```python
from build123d import *

# Parameters (mm, degrees)
SKETCH1_W           = 49.1
SKETCH1_H           = 80
BOSS_EXTRUDE1_DEPTH = 2
SKETCH2_R           = 1.7
CUT_EXTRUDE1_DEPTH  = 2
SKETCH3_W           = 5.2
SKETCH3_H           = 5.2
SKETCH3_R           = 1.7
BOSS_EXTRUDE2_DEPTH = 3.3
SKETCH4_W           = 7.5
SKETCH4_H           = 17.15
SKETCH4_W_2         = 5.1
CUT_EXTRUDE2_DEPTH  = 3.3
SKETCH7_W           = 38.7
SKETCH7_H           = 2.4
SKETCH7_W_2         = 2.4
SKETCH7_H_2         = 45.05
BOSS_EXTRUDE4_DEPTH = 3.3
SKETCH8_W           = 6.6
SKETCH8_H           = 1.2
SKETCH8_W_2         = 4.7
SKETCH8_H_2         = 6.2
BOSS_EXTRUDE5_DEPTH = 2.4
FILLET1_START       = -9.5
FILLET1_DEPTH       = 12.5
SKETCH9_R           = 2.5
CUT_EXTRUDE3_DEPTH  = 2
FILLET2_R           = 0.2


with BuildPart() as part:
    # Sketch1 → Boss-Extrude1 (new body)
    with BuildSketch(Plane(origin=(0, 0, 0), x_dir=(1, 0, 0), z_dir=(0, 1, 0))):
        with Locations((24.55, -40)):
            Rectangle(SKETCH1_W, SKETCH1_H)
    extrude(amount=BOSS_EXTRUDE1_DEPTH)

    # Sketch2 → Cut-Extrude1 (cut)
    with BuildSketch(Plane(origin=(0, 2, 0), x_dir=(1, 0, 0), z_dir=(0, 1, 0))):
        with Locations(Location((2.4, -77.6, 0), (0, 0, 270))):
            Circle(SKETCH2_R)
        with Locations(Location((2.45, -26.95, 0), (0, 0, 270))):
            Circle(SKETCH2_R)
        with Locations(Location((2.45, -5, 0), (0, 0, 270))):
            Circle(SKETCH2_R)
        with Locations(Location((46.7, -77.6, 0), (0, 0, 90))):
            Circle(SKETCH2_R)
        with Locations(Location((46.65, -26.95, 0), (0, 0, 90))):
            Circle(SKETCH2_R)
        with Locations(Location((46.65, -5, 0), (0, 0, 90))):
            Circle(SKETCH2_R)
    extrude(amount=-CUT_EXTRUDE1_DEPTH, mode=Mode.SUBTRACT)

    # Sketch3 → Boss-Extrude2 (add)
    # profile 1 of 6: a face of its own
    with BuildSketch(Plane.XZ):
        with Locations((2.6, 77.4)):
            Rectangle(SKETCH3_W, SKETCH3_H)
        with Locations(Location((2.4, 77.6, 0), (0, 0, 90))):
            Circle(SKETCH3_R, mode=Mode.SUBTRACT)
    # profile 2 of 6: a face of its own
    with BuildSketch(Plane.XZ):
        with Locations((2.6, 27.15)):
            Rectangle(SKETCH3_W, SKETCH3_H)
        with Locations(Location((2.45, 26.95, 0), (0, 0, 90))):
            Circle(SKETCH3_R, mode=Mode.SUBTRACT)
    # profile 3 of 6: a face of its own
    with BuildSketch(Plane.XZ):
        with Locations((2.6, 4.8)):
            Rectangle(SKETCH3_W, SKETCH3_H)
        with Locations(Location((2.45, 5, 0), (0, 0, 90))):
            Circle(SKETCH3_R, mode=Mode.SUBTRACT)
    # profile 4 of 6: a face of its own
    with BuildSketch(Plane.XZ):
        with Locations((46.5, 4.8)):
            Rectangle(SKETCH3_W, SKETCH3_H)
        with Locations(Location((46.65, 5, 0), (0, 0, 270))):
            Circle(SKETCH3_R, mode=Mode.SUBTRACT)
    # profile 5 of 6: a face of its own
    with BuildSketch(Plane.XZ):
        with Locations((46.5, 27.15)):
            Rectangle(SKETCH3_W, SKETCH3_H)
        with Locations(Location((46.65, 26.95, 0), (0, 0, 90))):
            Circle(SKETCH3_R, mode=Mode.SUBTRACT)
    # profile 6 of 6: a face of its own
    with BuildSketch(Plane.XZ):
        with Locations((46.5, 77.4)):
            Rectangle(SKETCH3_W, SKETCH3_H)
        with Locations(Location((46.7, 77.6, 0), (0, 0, 90))):
            Circle(SKETCH3_R, mode=Mode.SUBTRACT)
    extrude(amount=BOSS_EXTRUDE2_DEPTH)

    # Sketch4 → Cut-Extrude2 (cut)
    with BuildSketch(Plane(origin=(0, 2, 0), x_dir=(1, 0, 0), z_dir=(0, 1, 0))):
        with Locations((3.75, -15.975)):
            Rectangle(SKETCH4_W, SKETCH4_H)
        with Locations((46.55, -15.975)):
            Rectangle(SKETCH4_W_2, SKETCH4_H)
    extrude(amount=-CUT_EXTRUDE2_DEPTH, mode=Mode.SUBTRACT)

    # Sketch7 → Boss-Extrude4 (add)
    with BuildSketch(Plane.XZ):
        with Locations((24.55, 78.8)):
            Rectangle(SKETCH7_W, SKETCH7_H)
        with Locations((47.9, 52.275)):
            Rectangle(SKETCH7_W_2, SKETCH7_H_2)
        with Locations((1.2, 52.275)):
            Rectangle(SKETCH7_W_2, SKETCH7_H_2)
        Polygon((0, 0), (49.1, 0), (49.1, 2), (49.1, 2.2), (43.9, 2.2), (43.9, 2), (5.2, 2), (5.2, 2.2), (0, 2.2), (0, 2), align=None)
    extrude(amount=BOSS_EXTRUDE4_DEPTH)

    # Sketch8 → Boss-Extrude5 (add)
    with BuildSketch(Plane.XY.offset(80)):
        with Locations((27.8, -3.9)):
            Rectangle(SKETCH8_W, SKETCH8_H)
        with Locations((7.35, -6.4)):
            Rectangle(SKETCH8_W_2, SKETCH8_H_2)
    extrude(amount=-BOSS_EXTRUDE5_DEPTH)

    # Fillet1: read off the stored shape, not the designer's step
    # Fillet1 outline → Fillet1 (cut)
    with BuildSketch(Plane(origin=(0, 0, 0), x_dir=(1, 0, 0), z_dir=(0, 1, 0)).offset(FILLET1_START)):
        with BuildLine():
            Line((0, 0), (0, -2.4))
            ThreePointArc((0, -2.4), (0.702943725, -0.702943725), (2.4, 0))
            Line((2.4, 0), (0, 0))
        make_face()
        with BuildLine():
            ThreePointArc((2.4, -7.4), (0.702943725, -6.697056275), (0, -5))
            Line((0, -5), (0, -7.4))
            Line((0, -7.4), (2.4, -7.4))
        make_face()
        with BuildLine():
            Line((49.1, -7.4), (49.1, -5))
            ThreePointArc((49.1, -5), (48.397056275, -6.697056275), (46.7, -7.4))
            Line((46.7, -7.4), (49.1, -7.4))
        make_face()
        with BuildLine():
            Line((49.1, 0), (46.7, 0))
            ThreePointArc((46.7, 0), (48.397056275, -0.702943725), (49.1, -2.4))
            Line((49.1, -2.4), (49.1, 0))
        make_face()
        with BuildLine():
            Line((0, -80), (2.4, -80))
            ThreePointArc((2.4, -80), (0.702943725, -79.297056275), (0, -77.6))
            Line((0, -77.6), (0, -80))
        make_face()
        with BuildLine():
            ThreePointArc((46.7, -24.55), (48.397056275, -25.252943725), (49.1, -26.95))
            Line((49.1, -26.95), (49.1, -24.55))
            Line((49.1, -24.55), (46.7, -24.55))
        make_face()
        with BuildLine():
            ThreePointArc((49.1, -77.6), (48.397056275, -79.297056275), (46.7, -80))
            Line((46.7, -80), (49.1, -80))
            Line((49.1, -80), (49.1, -77.6))
        make_face()
        with BuildLine():
            Line((0, -24.55), (0, -26.95))
            ThreePointArc((0, -26.95), (0.702943725, -25.252943725), (2.4, -24.55))
            Line((2.4, -24.55), (0, -24.55))
        make_face()
    extrude(amount=FILLET1_DEPTH, mode=Mode.SUBTRACT)

    # Sketch9 → Cut-Extrude3 (cut)
    with BuildSketch(Plane(origin=(0, 2, 0), x_dir=(1, 0, 0), z_dir=(0, 1, 0))):
        with Locations((2.45, -5)):
            Circle(SKETCH9_R)
        with Locations((2.45, -26.95)):
            Circle(SKETCH9_R)
        with Locations((2.4, -77.6)):
            Circle(SKETCH9_R)
        with Locations((46.7, -77.6)):
            Circle(SKETCH9_R)
        with Locations((46.65, -26.95)):
            Circle(SKETCH9_R)
        with Locations((46.65, -5)):
            Circle(SKETCH9_R)
    extrude(amount=-CUT_EXTRUDE3_DEPTH, mode=Mode.SUBTRACT)

    # Fillet2
    fillet2_edges = [part.edges().sort_by_distance(p)[0] for p in [
        (45.95, 1, 24.55),
        (45.95, 1, 7.4),
        (3.15, 1, 7.4),
        (3.15, 1, 24.55),
        (49.1, 1, 4.502506281),
        (49.1, 1, 27.447493719),
        (49.1, 1, 76.9),
        (46, 1, 80),
        (0, 1, 76.9),
        (3.1, 1, 80),
        (0, 1, 27.447493719),
        (0, 1, 4.502506281),
    ]]
    fillet(fillet2_edges, radius=FILLET2_R)


solid = part.part
```
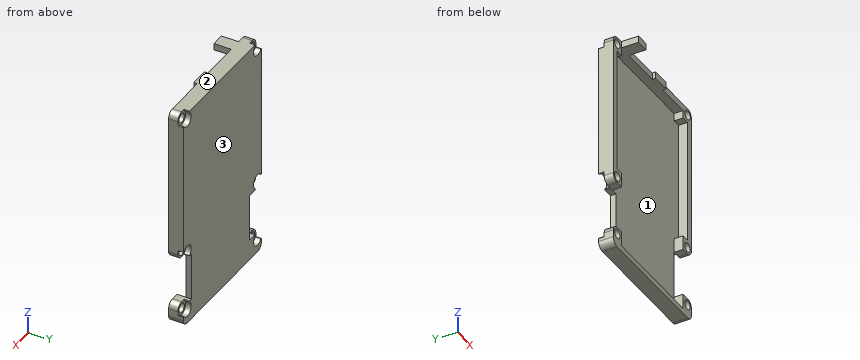
Work out the finished part from the listing and answer in its coordinate system (mm). Face numbers are marked on the shaded views. Round coordinates to 2 decimals unless told otherwise and drop trailing zeros. Loops run counter-clockwise (first coordinate to the right, second up) from the corner with the lowest first, then second, coordinate; pieces in that order, holes last. Notation, with made-up numbers: M 12.5,69 L 23.5,69 A10 ccw 23.5,76 Z; hole C 79.25,-5.75 d7. An arc over 180 degrees is marked long. One line per question, with ' | ' between items.
Q1. Find section D-D, the plane y = -8.25. Give the vertices of the cut face in (x, z), then the cut area to 3 significant figures.
Conclusion:
outline: M 5,77.6 L 9.7,77.6 L 9.7,80 L 5,80 Z | area: 11.3 mm2
Q2. Find section C-C, the plane y = -1. State how many separate pieces and enclosed holes the cut face has, then the cut area to 3 significant figures.
Conclusion:
separate pieces: 2 | enclosed holes: 6 | area: 507 mm2
Q3. Each of these flat-tipped pins is pushed along its axis until it touches: pin 1 Ø2.5 at (y, z) = (-7.5, 78.5) entering from +X; pin 2 Ø4.5 at (x, z) = (46.65, 5) entering from -Y; pin 3 Ø4 at (x, y) = (9.5, -5.5) entering from -Z. Where does it stop, or does it pass through?
Conclusion:
pin 1: stops at x = 9.7 | pin 2: stops at y = -3.3 | pin 3: stops at z = 77.6
Q4. Find section A-A, the plane x = 17.5. Give the vertices of the cut face in (y, z), then the cut area to 3 significant figures.
Conclusion:
outline: M -3.3,0 L 2,0 L 2,80 L -3.3,80 L -3.3,77.6 L 0,77.6 L 0,2 L -3.3,2 Z | area: 175 mm2
Q5. Find section B-B, the plane z = 52. Give the vertices of the cut face in (x, y).
Conclusion:
outline: M 0,-3.3 L 2.4,-3.3 L 2.4,0 L 46.7,0 L 46.7,-3.3 L 49.1,-3.3 L 49.1,2 L 0,2 Z
Q6. Consider line 1 along X through (y, z) = (-2.1, 5); line 2 along Z through (x, y) = (18.5, -2.5); line 3 along X through (y, z) = (-3, 73). Determine where each line is inside the solid, lowest interval first. Write a range as from..to.
Conclusion:
line 1: x = 0..0.75, 4.15..5.2, 43.9..44.95, 48.35..49.1 | line 2: z = 0..2, 77.6..80 | line 3: x = 0..2.4, 46.7..49.1
Q7. The mould has two halves that part along Z. Classify the marked faces 1, 2 and 3: +Z half, -Z half, draft (parallel to the pull), parting line (faces both ways), or undercut.
Conclusion:
face 1: undercut | face 2: +Z half | face 3: draft
